Check sheet for the modelled part. Datum: model origin and axes. Units: mm. Round coordinates to 2 decimals unless told otherwise and drop trailing zeros. Loops run counter-clockwise (first coordinate to the right, second up) from the corner with the lowest first, then second, coordinate; pieces in that order, holes last. Notation, with made-up numbers: (82, -24.5) - (131, -24.5) arc R27 cw to (131, 2.5) - close; hole circle Ø11 at (75, 39). An arc over 180 degrees is marked (long way). Return JSON: item names as keys, results as strings.
from build123d import *

# Parameters (mm, degrees)
SKETCH1_W           = 0.79375
SKETCH1_H           = 19.05
SKETCH1_R           = 1.5875
BOSS_EXTRUDE1_DEPTH = 3.175


with BuildPart() as part:
    # Sketch1 → Boss-Extrude1 (new body)
    with BuildSketch(Plane.XY.offset(-196.85)):
        with BuildLine():
            Line((-85.725, -136.525), (-94.488, -136.525))
            Line((-94.488, -136.525), (-94.488, -171.45))
            ThreePointArc((-94.488, -171.45), (-87.271696875, -188.871696875), (-69.85, -196.088))
            Line((-69.85, -196.088), (-50.8, -196.088))
            Line((-50.8, -196.088), (-50.8, -192.913))
            Line((-50.8, -192.913), (-25.4, -192.913))
            Line((-25.4, -192.913), (-25.4, -196.088))
            Line((-25.4, -196.088), (25.4, -196.088))
            Line((25.4, -196.088), (25.4, -192.913))
            Line((25.4, -192.913), (50.8, -192.913))
            Line((50.8, -192.913), (50.8, -196.088))
            Line((50.8, -196.088), (69.85, -196.088))
            ThreePointArc((69.85, -196.088), (87.271696875, -188.871696875), (94.488, -171.45))
            Line((94.488, -171.45), (94.488, -136.525))
            Line((94.488, -136.525), (85.725, -136.525))
            Line((85.725, -136.525), (85.725, -115.57))
            ThreePointArc((85.725, -115.57), (85.353025612, -114.671974388), (84.455, -114.3))
            Line((84.455, -114.3), (63.5, -114.3))
            Line((63.5, -114.3), (63.5, -111.125))
            Line((63.5, -111.125), (94.488, -111.125))
            Line((94.488, -111.125), (94.488, -85.725))
            Line((94.488, -85.725), (88.9, -85.725))
            Line((88.9, -85.725), (88.9, -60.325))
            Line((88.9, -60.325), (94.488, -60.325))
            Line((94.488, -60.325), (94.488, -25.4))
            ThreePointArc((94.488, -25.4), (87.271696875, -7.978303125), (69.85, -0.762))
            Line((69.85, -0.762), (-69.85, -0.762))
            ThreePointArc((-69.85, -0.762), (-87.271696875, -7.978303125), (-94.488, -25.4))
            Line((-94.488, -25.4), (-94.488, -60.325))
            Line((-94.488, -60.325), (-88.9, -60.325))
            Line((-88.9, -60.325), (-88.9, -85.725))
            Line((-88.9, -85.725), (-94.488, -85.725))
            Line((-94.488, -85.725), (-94.488, -111.125))
            Line((-94.488, -111.125), (-63.5, -111.125))
            Line((-63.5, -111.125), (-63.5, -114.3))
            Line((-63.5, -114.3), (-84.455, -114.3))
            ThreePointArc((-84.455, -114.3), (-85.353025612, -114.671974388), (-85.725, -115.57))
            Line((-85.725, -115.57), (-85.725, -136.525))
        make_face()
        with Locations((-89.296875, -158.75)):
            Rectangle(SKETCH1_W, SKETCH1_H, mode=Mode.SUBTRACT)
        with BuildLine():
            ThreePointArc((-69.85, -173.0375), (-71.4375, -171.45), (-69.85, -169.8625))
            Line((-69.85, -169.8625), (-60.325, -169.8625))
            ThreePointArc((-60.325, -169.8625), (-58.7375, -171.45), (-60.325, -173.0375))
            Line((-60.325, -173.0375), (-69.85, -173.0375))
        make_face(mode=Mode.SUBTRACT)
        with Locations((-19.05, -159.40600326)):
            Circle(SKETCH1_R, mode=Mode.SUBTRACT)
        with Locations((-19.05, -130.83100326)):
            Circle(SKETCH1_R, mode=Mode.SUBTRACT)
        with Locations((19.05, -159.40600326)):
            Circle(SKETCH1_R, mode=Mode.SUBTRACT)
        with Locations((69.85, -171.45)):
            Circle(SKETCH1_R, mode=Mode.SUBTRACT)
        with Locations((89.296875, -158.75)):
            Rectangle(SKETCH1_W, SKETCH1_H, mode=Mode.SUBTRACT)
        with Locations((19.05, -130.83100326)):
            Circle(SKETCH1_R, mode=Mode.SUBTRACT)
        with BuildLine():
            ThreePointArc((-67.060192091, -72.204012806), (-69.124952547, -69.113880409), (-69.85, -65.468820715))
            Line((-69.85, -65.468820715), (-69.85, -40.839204897))
            ThreePointArc((-69.85, -40.839204897), (-66.714031836, -36.145896872), (-61.177897552, -37.247102448))
            Line((-61.177897552, -37.247102448), (-18.197102448, -80.227897552))
            ThreePointArc((-18.197102448, -80.227897552), (-17.095896872, -85.764031836), (-21.789204897, -88.9))
            Line((-21.789204897, -88.9), (-46.418820715, -88.9))
            ThreePointArc((-46.418820715, -88.9), (-50.063880409, -88.174952547), (-53.154012806, -86.110192091))
            Line((-53.154012806, -86.110192091), (-67.060192091, -72.204012806))
        make_face(mode=Mode.SUBTRACT)
        with Locations((-69.85, -25.4)):
            Circle(SKETCH1_R, mode=Mode.SUBTRACT)
        with Locations((-19.05, -12.7)):
            Circle(SKETCH1_R, mode=Mode.SUBTRACT)
        with BuildLine():
            ThreePointArc((3.592102448, -81.36251337), (0, -82.850410922), (-3.592102448, -81.36251337))
            Line((-3.592102448, -81.36251337), (-50.88251337, -34.072102448))
            ThreePointArc((-50.88251337, -34.072102448), (-51.983718947, -28.535968164), (-47.290410922, -25.4))
            Line((-47.290410922, -25.4), (47.290410922, -25.4))
            ThreePointArc((47.290410922, -25.4), (51.983718947, -28.535968164), (50.88251337, -34.072102448))
            Line((50.88251337, -34.072102448), (3.592102448, -81.36251337))
        make_face(mode=Mode.SUBTRACT)
        with BuildLine():
            ThreePointArc((53.154012806, -86.110192091), (50.063880409, -88.174952547), (46.418820715, -88.9))
            Line((46.418820715, -88.9), (21.789204897, -88.9))
            ThreePointArc((21.789204897, -88.9), (17.095896872, -85.764031836), (18.197102448, -80.227897552))
            Line((18.197102448, -80.227897552), (61.177897552, -37.247102448))
            ThreePointArc((61.177897552, -37.247102448), (66.714031836, -36.145896872), (69.85, -40.839204897))
            Line((69.85, -40.839204897), (69.85, -65.468820715))
            ThreePointArc((69.85, -65.468820715), (69.124952547, -69.113880409), (67.060192091, -72.204012806))
            Line((67.060192091, -72.204012806), (53.154012806, -86.110192091))
        make_face(mode=Mode.SUBTRACT)
        with Locations((19.05, -12.7)):
            Circle(SKETCH1_R, mode=Mode.SUBTRACT)
        with Locations((69.85, -25.4)):
            Circle(SKETCH1_R, mode=Mode.SUBTRACT)
    extrude(amount=-BOSS_EXTRUDE1_DEPTH)


solid = part.part
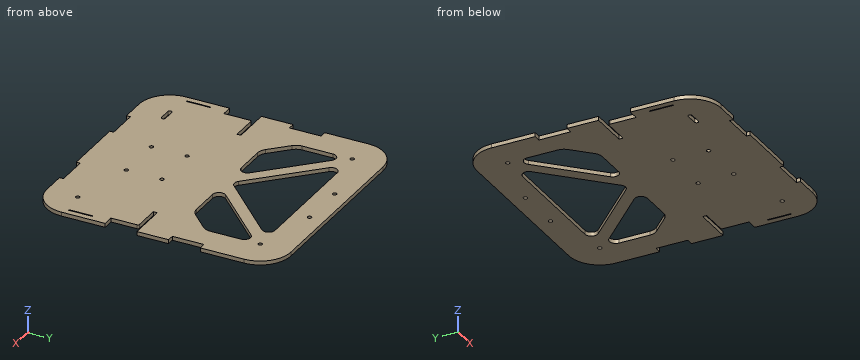
Q1. Depth check by flat-ended pin: P1, Ø1.6, axis at x = -35, z = -198, coming from the -Y side; P2, Ø1.5, axis at y = -123.5, z = -199.5, coming from the -X side (3 decimals); P3, Ø2.5, axis at x = 19.05, y = -159.41, coming from the +Z side. Enter the tip coordinate at first touch or a pass-through.
Answer key:
{"P1": "stops at y = -192.91", "P2": "stops at x = -85.725", "P3": "passes through"}
Q2. Sectioned sample at D-D (z = -197.35). State how many separate pieces and enclosed holes the cut face has, plus the area to 3 significant figures.
Answer key:
{"separate pieces": "1", "enclosed holes": "15", "area": "28,600 mm²"}
Q3. Sectioned sample at A-A (x = 7). Enter the section's corners in (y, z) (3 decimals).
Answer key:
{"outline": "(-196.088, -200.025) - (-77.955, -200.025) - (-77.955, -196.85) - (-196.088, -196.85) - close; (-25.4, -200.025) - (-0.762, -200.025) - (-0.762, -196.85) - (-25.4, -196.85) - close"}
Q4. Scan lines: probe 1 along Y at (x, z) = (34, -199) (3 decimals); probe 2 along Y at (x, z) = (19.05, -199.2) (1 decimal); probe 3 along Y at (x, z) = (22.5, -199.6) (3 decimals). Record each from-to range of solid material in increasing order. Write a range as [from, to].
Answer key:
{"probe 1": "y = [-192.913, -88.9], [-64.425, -50.955], [-25.4, -0.762]", "probe 2": "y = [-196.1, -161], [-157.8, -132.4], [-129.2, -88.1], [-79.4, -65.9], [-25.4, -14.3], [-11.1, -0.8]", "probe 3": "y = [-196.088, -88.9], [-75.925, -62.455], [-25.4, -0.762]"}
Q5. Sectioned sample at B-B (y = -44.5). Enter the section's corners in (x, z) (3 decimals), plus the area to 3 significant figures.
Answer key:
{"outline": "(-94.488, -200.025) - (-69.85, -200.025) - (-69.85, -196.85) - (-94.488, -196.85) - close; (-53.925, -200.025) - (-40.455, -200.025) - (-40.455, -196.85) - (-53.925, -196.85) - close; (40.455, -200.025) - (53.925, -200.025) - (53.925, -196.85) - (40.455, -196.85) - close; (69.85, -200.025) - (94.488, -200.025) - (94.488, -196.85) - (69.85, -196.85) - close", "area": "242 mm²"}
Q6. Sectioned sample at C-C (x = -77). Enter the section's corners in (y, z) (3 decimals).
Answer key:
{"outline": "(-195.028, -200.025) - (-114.3, -200.025) - (-114.3, -196.85) - (-195.028, -196.85) - close; (-111.125, -200.025) - (-1.822, -200.025) - (-1.822, -196.85) - (-111.125, -196.85) - close"}
